Part model, mm, in its own coordinate system. Face numbers are marked on the shaded views. Coordinates: 2 decimals unless noted, no trailing zeros. Loops run counter-clockwise (first coordinate to the right, second up) from the corner with the lowest first, then second, coordinate; pieces in that order, holes last. Notation, with made-up numbers: M 85.5,-30 L 103.5,-30 A22 ccw 103.5,-24 Z; hole C 23.5,81 d9. An arc over 180 degrees is marked long. Answer as a JSON object with one key per item and string values. Group by question number.
1. Drop flat-ended pins along their axis: pin 1 Ø1 at (x, z) = (2.5, 1.5) entering from -Y; pin 2 Ø1.5 at (x, y) = (-2.5, -61.5) entering from -Z. Give the stop position or say it passes through.
2. Saw through at A-A on x = 0. Write the cut outline in (y, z) (1 decimal), then the cut area to 3 significant figures.
3. Drill centre lines: L1, parallel to Z at x = -2.5, y = -3; L2, parallel to Y at x = -1.25, z = -4.5; L3, parallel to X at y = -1.5, z = -7. Where is each one in solid material? Low to high.
4. Mould opens along Y. For the marked faces 1 and 2 say: released by +Y, released by -Y, zero draft, split by the parting line, or undercut.
5. Saw through at C-C on y = -35. Write the cut outline in (x, z) (3 decimals), then the cut area to 3 significant figures.
from build123d import *

# Parameters (mm, degrees)
SKETCH1_R           = 1.5875
BOSS_EXTRUDE1_DEPTH = 2.54
BOSS_EXTRUDE2_START = -10.16
SKETCH2_R           = 1.72979554
SKETCH2_R_2         = 1.5875
BOSS_EXTRUDE2_DEPTH = 10.16


with BuildPart() as part:
    # Sketch1 → Boss-Extrude1 (new body)
    with BuildSketch(Plane.XY):
        with BuildLine():
            Line((-3.175, 0), (-3.175, -95.25))
            ThreePointArc((-3.175, -95.25), (0, -98.425), (3.175, -95.25))
            Line((3.175, -95.25), (3.175, 0))
            ThreePointArc((3.175, 0), (0, 3.175), (-3.175, 0))
        make_face()
        Circle(SKETCH1_R, mode=Mode.SUBTRACT)
        with Locations((0, -95.25)):
            Circle(SKETCH1_R, mode=Mode.SUBTRACT)
    extrude(amount=BOSS_EXTRUDE1_DEPTH)

    # Sketch2 → Boss-Extrude2 (add)
    with BuildSketch(Plane.XY.offset(2.54).offset(BOSS_EXTRUDE2_START)):
        Circle(SKETCH2_R)
        with Locations((0, -95.25)):
            Circle(SKETCH2_R_2)
    extrude(amount=BOSS_EXTRUDE2_DEPTH)


solid = part.part
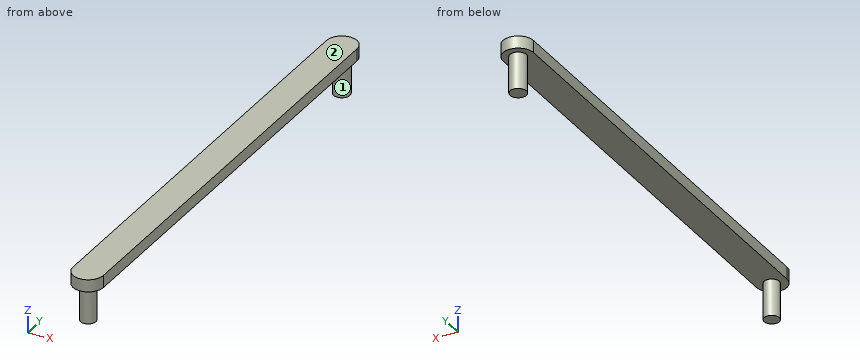
Outcome:
{
 "1": {"pin 1": "stops at y = -97.72", "pin 2": "stops at z = 0"},
 "2": {"outline": "M -98.4,0 L -96.8,0 L -96.8,-7.6 L -93.7,-7.6 L -93.7,0 L -1.7,0 L -1.7,-7.6 L 1.7,-7.6 L 1.7,0 L 3.2,0 L 3.2,2.5 L -98.4,2.5 Z", "area": "309 mm²"},
 "3": {"L1": "z = 0 to 2.54", "L2": "y = -96.23 to -94.27, -1.2 to 1.2", "L3": "x = -0.86 to 0.86"},
 "4": {"face 1": "undercut", "face 2": "zero draft"},
 "5": {"outline": "M -3.175,0 L 3.175,0 L 3.175,2.54 L -3.175,2.54 Z", "area": "16.1 mm²"}
}
